Source: CAD feature listing. Evaluate the final solid. Frame: model axes, mm. Give positions to 0.01 mm unless a question says otherwise; leave off trailing zeros.
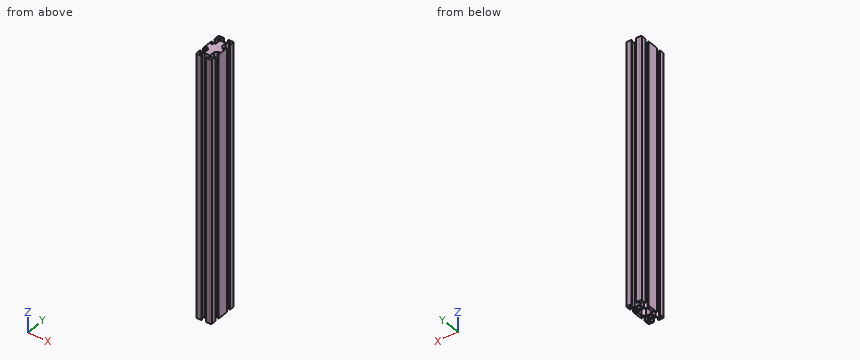
from build123d import *

# Parameters (mm, degrees)
EXTRUSION2_DEPTH           = 161.5
EXTRUSION2_DEPTH_BACK      = 161.5
SKETCH1_R                  = 3.25
F_4_7_4_7_DIAMETER_HOLE1_D = 4.75
BOSS_EXTRUDE1_DEPTH        = 150


with BuildPart() as part:
    # Sketch1 → Extrusion2 (new, two sides: drawn at the far end of the back side and taken through both)
    with BuildSketch(Plane.XY.offset(-EXTRUSION2_DEPTH_BACK)):
        with BuildLine():
            Line((-51.945456549, 19.536039976), (-51.945456549, -0.463960024))
            Line((-51.945456549, -0.463960024), (-49.945456549, -0.463960024))
            Line((-49.945456549, -0.463960024), (-49.945456549, 4.741263919))
            Line((-49.945456549, 4.741263919), (-48.386244669, 4.741263919))
            Line((-48.386244669, 4.741263919), (-43.445456549, -0.1995242))
            Line((-43.445456549, -0.1995242), (-43.445456549, -8.717947961))
            Line((-43.445456549, -8.717947961), (-48.386244669, -13.658736081))
            Line((-48.386244669, -13.658736081), (-49.945456549, -13.658736081))
            Line((-49.945456549, -13.658736081), (-49.945456549, -8.458736081))
            Line((-49.945456549, -8.458736081), (-51.945456549, -8.458736081))
            Line((-51.945456549, -8.458736081), (-51.945456549, -16.458736081))
            ThreePointArc((-51.945456549, -16.458736081), (-51.359670111, -17.872949643), (-49.945456549, -18.458736081))
            Line((-49.945456549, -18.458736081), (-41.945456549, -18.458736081))
            Line((-41.945456549, -18.458736081), (-41.945456549, -16.458736081))
            Line((-41.945456549, -16.458736081), (-47.145456549, -16.458736081))
            Line((-47.145456549, -16.458736081), (-47.145456549, -14.8995242))
            Line((-47.145456549, -14.8995242), (-42.204668429, -9.958736081))
            Line((-42.204668429, -9.958736081), (-33.686244669, -9.958736081))
            Line((-33.686244669, -9.958736081), (-28.745456549, -14.8995242))
            Line((-28.745456549, -14.8995242), (-28.745456549, -16.458736081))
            Line((-28.745456549, -16.458736081), (-33.945456549, -16.458736081))
            Line((-33.945456549, -16.458736081), (-33.945456549, -18.458736081))
            Line((-33.945456549, -18.458736081), (-25.945456549, -18.458736081))
            ThreePointArc((-25.945456549, -18.458736081), (-24.531242987, -17.872949643), (-23.945456549, -16.458736081))
            Line((-23.945456549, -16.458736081), (-23.945456549, -8.458736081))
            Line((-23.945456549, -8.458736081), (-25.945456549, -8.458736081))
            Line((-25.945456549, -8.458736081), (-25.945456549, -13.658736081))
            Line((-25.945456549, -13.658736081), (-27.504668429, -13.658736081))
            Line((-27.504668429, -13.658736081), (-32.445456549, -8.717947961))
            Line((-32.445456549, -8.717947961), (-32.445456549, -0.1995242))
            Line((-32.445456549, -0.1995242), (-27.504668429, 4.741263919))
            Line((-27.504668429, 4.741263919), (-25.945456549, 4.741263919))
            Line((-25.945456549, 4.741263919), (-25.945456549, -0.463960024))
            Line((-25.945456549, -0.463960024), (-23.945456549, -0.463960024))
            Line((-23.945456549, -0.463960024), (-23.945456549, 19.541263919))
            Line((-23.945456549, 19.541263919), (-25.945456549, 19.541263919))
            Line((-25.945456549, 19.541263919), (-25.945456549, 14.341263919))
            Line((-25.945456549, 14.341263919), (-27.504668429, 14.341263919))
            Line((-27.504668429, 14.341263919), (-32.445456549, 19.282052039))
            Line((-32.445456549, 19.282052039), (-32.445456549, 27.8004758))
            Line((-32.445456549, 27.8004758), (-27.504668429, 32.741263919))
            Line((-27.504668429, 32.741263919), (-25.945456549, 32.741263919))
            Line((-25.945456549, 32.741263919), (-25.945456549, 27.541263919))
            Line((-25.945456549, 27.541263919), (-23.945456549, 27.541263919))
            Line((-23.945456549, 27.541263919), (-23.945456549, 35.541263919))
            ThreePointArc((-23.945456549, 35.541263919), (-24.531242987, 36.955477482), (-25.945456549, 37.541263919))
            Line((-25.945456549, 37.541263919), (-33.945456549, 37.541263919))
            Line((-33.945456549, 37.541263919), (-33.945456549, 35.541263919))
            Line((-33.945456549, 35.541263919), (-28.745456549, 35.541263919))
            Line((-28.745456549, 35.541263919), (-28.745456549, 33.982052039))
            Line((-28.745456549, 33.982052039), (-33.686244669, 29.041263919))
            Line((-33.686244669, 29.041263919), (-42.204668429, 29.041263919))
            Line((-42.204668429, 29.041263919), (-47.145456549, 33.982052039))
            Line((-47.145456549, 33.982052039), (-47.145456549, 35.541263919))
            Line((-47.145456549, 35.541263919), (-41.945456549, 35.541263919))
            Line((-41.945456549, 35.541263919), (-41.945456549, 37.541263919))
            Line((-41.945456549, 37.541263919), (-49.945456549, 37.541263919))
            ThreePointArc((-49.945456549, 37.541263919), (-51.359670111, 36.955477482), (-51.945456549, 35.541263919))
            Line((-51.945456549, 35.541263919), (-51.945456549, 27.541263919))
            Line((-51.945456549, 27.541263919), (-49.945456549, 27.541263919))
            Line((-49.945456549, 27.541263919), (-49.945456549, 32.736039976))
            Line((-49.945456549, 32.736039976), (-48.372120999, 32.736039976))
            Line((-48.372120999, 32.736039976), (-43.43133288, 27.795251856))
            Line((-43.43133288, 27.795251856), (-43.43133288, 19.276828096))
            Line((-43.43133288, 19.276828096), (-48.372120999, 14.336039976))
            Line((-48.372120999, 14.336039976), (-49.93133288, 14.336039976))
            Line((-49.93133288, 14.336039976), (-49.93133288, 19.536039976))
            Line((-49.93133288, 19.536039976), (-51.945456549, 19.536039976))
        make_face()
        with Locations((-37.945456549, -4.458736081)):
            Circle(SKETCH1_R, mode=Mode.SUBTRACT)
        with Locations((-37.945456549, 23.541263919)):
            Circle(SKETCH1_R, mode=Mode.SUBTRACT)
        Polygon((-33.686244669, 18.041263919), (-42.204668429, 18.041263919), (-47.145456549, 13.1004758), (-47.145456549, 5.982052039), (-42.204668429, 1.041263919), (-33.686244669, 1.041263919), (-28.745456549, 5.982052039), (-28.745456549, 13.1004758), align=None, mode=Mode.SUBTRACT)
    extrude(amount=EXTRUSION2_DEPTH + EXTRUSION2_DEPTH_BACK)

    # Ø4.7 (4.7) Diameter Hole1 (through all)
    with Locations(Plane(origin=(-23.945456549, 0, 0), x_dir=(0, 0, -1), z_dir=(1, 0, 0))):
        with Locations((-140.5, 23.541263919), (140.5, 23.541263919)):
            Hole(F_4_7_4_7_DIAMETER_HOLE1_D / 2)

    # Sketch5 → Boss-Extrude1 (add)
    with BuildSketch(Plane.XY.offset(161.5)):
        with BuildLine():
            Line((-41.945456549, 37.541263919), (-49.945456549, 37.541263919))
            ThreePointArc((-49.945456549, 37.541263919), (-51.359670111, 36.955477482), (-51.945456549, 35.541263919))
            Line((-51.945456549, 35.541263919), (-51.945456549, 27.541263919))
            Line((-51.945456549, 27.541263919), (-49.945456549, 27.541263919))
            Line((-49.945456549, 27.541263919), (-49.945456549, 32.736039976))
            Line((-49.945456549, 32.736039976), (-48.372120999, 32.736039976))
            Line((-48.372120999, 32.736039976), (-43.43133288, 27.795251856))
            Line((-43.43133288, 27.795251856), (-43.43133288, 19.276828096))
            Line((-43.43133288, 19.276828096), (-48.372120999, 14.336039976))
            Line((-48.372120999, 14.336039976), (-49.93133288, 14.336039976))
            Line((-49.93133288, 14.336039976), (-49.93133288, 19.536039976))
            Line((-49.93133288, 19.536039976), (-51.945456549, 19.536039976))
            Line((-51.945456549, 19.536039976), (-51.945456549, -0.463960024))
            Line((-51.945456549, -0.463960024), (-49.945456549, -0.463960024))
            Line((-49.945456549, -0.463960024), (-49.945456549, 4.741263919))
            Line((-49.945456549, 4.741263919), (-48.386244669, 4.741263919))
            Line((-48.386244669, 4.741263919), (-43.445456549, -0.1995242))
            Line((-43.445456549, -0.1995242), (-43.445456549, -8.717947961))
            Line((-43.445456549, -8.717947961), (-48.386244669, -13.658736081))
            Line((-48.386244669, -13.658736081), (-49.945456549, -13.658736081))
            Line((-49.945456549, -13.658736081), (-49.945456549, -8.458736081))
            Line((-49.945456549, -8.458736081), (-51.945456549, -8.458736081))
            Line((-51.945456549, -8.458736081), (-51.945456549, -16.458736081))
            ThreePointArc((-51.945456549, -16.458736081), (-51.359670111, -17.872949643), (-49.945456549, -18.458736081))
            Line((-49.945456549, -18.458736081), (-41.945456549, -18.458736081))
            Line((-41.945456549, -18.458736081), (-41.945456549, -16.458736081))
            Line((-41.945456549, -16.458736081), (-47.145456549, -16.458736081))
            Line((-47.145456549, -16.458736081), (-47.145456549, -14.8995242))
            Line((-47.145456549, -14.8995242), (-42.204668429, -9.958736081))
            Line((-42.204668429, -9.958736081), (-33.686244669, -9.958736081))
            Line((-33.686244669, -9.958736081), (-28.745456549, -14.8995242))
            Line((-28.745456549, -14.8995242), (-28.745456549, -16.458736081))
            Line((-28.745456549, -16.458736081), (-33.945456549, -16.458736081))
            Line((-33.945456549, -16.458736081), (-33.945456549, -18.458736081))
            Line((-33.945456549, -18.458736081), (-25.945456549, -18.458736081))
            ThreePointArc((-25.945456549, -18.458736081), (-24.531242987, -17.872949643), (-23.945456549, -16.458736081))
            Line((-23.945456549, -16.458736081), (-23.945456549, -8.458736081))
            Line((-23.945456549, -8.458736081), (-25.945456549, -8.458736081))
            Line((-25.945456549, -8.458736081), (-25.945456549, -13.658736081))
            Line((-25.945456549, -13.658736081), (-27.504668429, -13.658736081))
            Line((-27.504668429, -13.658736081), (-32.445456549, -8.717947961))
            Line((-32.445456549, -8.717947961), (-32.445456549, -0.1995242))
            Line((-32.445456549, -0.1995242), (-27.504668429, 4.741263919))
            Line((-27.504668429, 4.741263919), (-25.945456549, 4.741263919))
            Line((-25.945456549, 4.741263919), (-25.945456549, -0.463960024))
            Line((-25.945456549, -0.463960024), (-23.945456549, -0.463960024))
            Line((-23.945456549, -0.463960024), (-23.945456549, 19.541263919))
            Line((-23.945456549, 19.541263919), (-25.945456549, 19.541263919))
            Line((-25.945456549, 19.541263919), (-25.945456549, 14.341263919))
            Line((-25.945456549, 14.341263919), (-27.504668429, 14.341263919))
            Line((-27.504668429, 14.341263919), (-32.445456549, 19.282052039))
            Line((-32.445456549, 19.282052039), (-32.445456549, 27.8004758))
            Line((-32.445456549, 27.8004758), (-27.504668429, 32.741263919))
            Line((-27.504668429, 32.741263919), (-25.945456549, 32.741263919))
            Line((-25.945456549, 32.741263919), (-25.945456549, 27.541263919))
            Line((-25.945456549, 27.541263919), (-23.945456549, 27.541263919))
            Line((-23.945456549, 27.541263919), (-23.945456549, 35.541263919))
            ThreePointArc((-23.945456549, 35.541263919), (-24.531242987, 36.955477482), (-25.945456549, 37.541263919))
            Line((-25.945456549, 37.541263919), (-33.945456549, 37.541263919))
            Line((-33.945456549, 37.541263919), (-33.945456549, 35.541263919))
            Line((-33.945456549, 35.541263919), (-28.745456549, 35.541263919))
            Line((-28.745456549, 35.541263919), (-28.745456549, 33.982052039))
            Line((-28.745456549, 33.982052039), (-33.686244669, 29.041263919))
            Line((-33.686244669, 29.041263919), (-42.204668429, 29.041263919))
            Line((-42.204668429, 29.041263919), (-47.145456549, 33.982052039))
            Line((-47.145456549, 33.982052039), (-47.145456549, 35.541263919))
            Line((-47.145456549, 35.541263919), (-41.945456549, 35.541263919))
            Line((-41.945456549, 35.541263919), (-41.945456549, 37.541263919))
        make_face()
    extrude(amount=BOSS_EXTRUDE1_DEPTH)


solid = part.part
1) First-contact query: pin 1 Ø5 at (x, z) = (-37, 206.5) entering from +Y; pin 2 Ø2 at (y, z) = (36, 52.5) entering from -X; pin 3 Ø5 at (y, z) = (24.5, 70) entering from -X; pin 4 Ø5 at (x, y) = (-36.5, 10.5) entering from -Z. Flat tips, straight axial feed; report the tip coordinate or a pass-through.
Checks:
pin 1: stops at y = 29.04
pin 2: stops at x = -51.95
pin 3: stops at x = -43.43
pin 4: stops at z = 161.5
2) Ray query, L1, parallel to Y at x = -33.75, z = -43; L2, parallel to Y at x = -49.75, z = -17.5; L3, parallel to Y at x = -37.25, z = 18. Return the intervals inside material, ascending.
Checks:
L1: y = -18.46 to -16.46, -9.96 to 1.04, 18.04 to 29.04, 35.54 to 37.54
L2: y = -18.46 to -13.66, 4.74 to 14.34, 32.74 to 37.54
L3: y = -9.96 to -7.63, -1.28 to 1.04, 18.04 to 20.37, 26.72 to 29.04
3) Section query A-A on z = -54. State how many separate pieces and enclosed holes the cut face has, and give its area (3 significant figures).
Checks:
separate pieces: 1
enclosed holes: 3
area: 567 mm2
